The drawing under review shows one solid part. Ordinate dimensions are in mm from its lowest x, y, z. Give positions to 0.01 mm unless a question says otherwise; leave off trailing zeros. Write each loop counter-clockwise with the first axis right and the second up, starting at its lowest first coordinate (ties: lowest second). Pieces come first, ordered by that corner, then holes. Notation, with made-up numbers: (25.5, 64.5) -> (30.5, 64.5) arc R18 ccw to (30.5, 87.5) -> close; hole circle Ø5 at (28, 54.25). An arc over 180 degrees is marked (long way). Use CSV: the item, a comma, the result in double quotes.
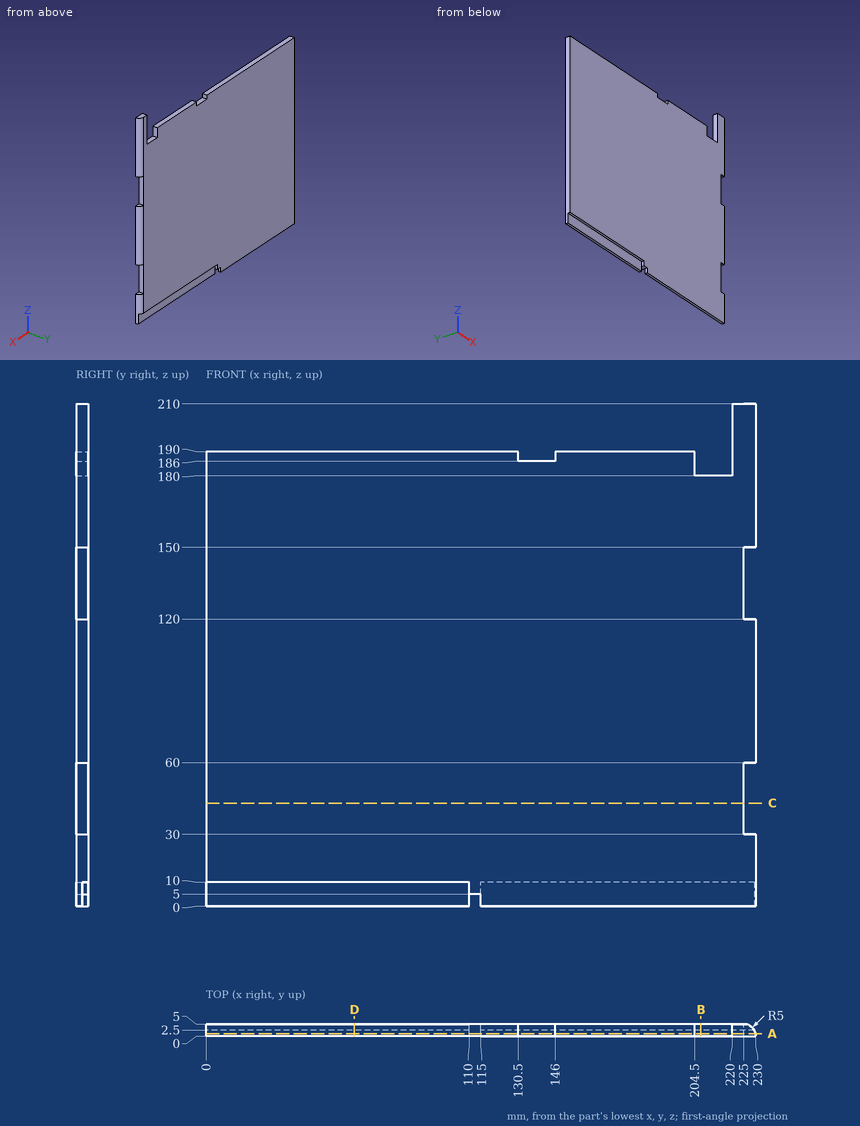
(1) Take a section at B-B (x = 207). Write out the cut boundary in (y, z), then the cut area to 3 significant figures.
Established:
outline,"(0, 0) -> (2.5, 0) -> (2.5, 10) -> (5, 10) -> (5, 180) -> (0, 180) -> close"
area,"875 mm2"
(2) Clearance check with flat-ended pins moving along their axes: pin 1 (8 mm diameter, centred on x = 132.5, z = 166, fed in from -Y); pin 2 (1 mm diameter, centred on x = 123.5, y = 1, fed in from +Z); pin 3 (2 mm diameter, centred on y = 1.5, z = 188.5, fed in from +X) (3 decimals); pin 4 (3 mm diameter, centred on x = 51.5, y = 0.5, fed in from -Z). State where each tip first meets the part, or that it passes through.
Established:
pin 1,"stops at y = 0"
pin 2,"stops at z = 190"
pin 3,"stops at x = 229.975"
pin 4,"stops at z = 10"
(3) Take a section at D-D (x = 62). Write out the cut boundary in (y, z), then the cut area to 3 significant figures.
Established:
outline,"(0, 10) -> (2.5, 10) -> (2.5, 0) -> (5, 0) -> (5, 190) -> (0, 190) -> close"
area,"925 mm2"
(4) Take a section at A-A (y = 0.95). Write out the cut boundary in (x, z), then the cut area to 3 significant figures.
Established:
outline,"(0, 10) -> (110, 10) -> (110, 5) -> (115, 5) -> (115, 0) -> (229.91, 0) -> (229.91, 30) -> (225, 30) -> (225, 60) -> (229.91, 60) -> (229.91, 120) -> (225, 120) -> (225, 150) -> (229.91, 150) -> (229.91, 210) -> (220, 210) -> (220, 180) -> (204.5, 180) -> (204.5, 190) -> (146, 190) -> (146, 186) -> (130.5, 186) -> (130.5, 190) -> (0, 190) -> close"
area,"42,200 mm2"
(5) Take a section at C-C (z = 43). Write out the cut boundary in (x, y), then the cut area to 4 significant figures.
Established:
outline,"(0, 0) -> (225, 0) -> (225, 5) -> (0, 5) -> close"
area,"1,125 mm2"
(6) For line 1 along X through (y, z) = (1.45, 189) (3 decimals); line 2 along X through (y, z) = (4.3, 120.5); line 3 along X through (y, z) = (0.25, 68.5), list the stretches that pass through material, from the lowest coordinate up. Write a range as [from, to].
Established:
line 1,"x = [0, 130.5], [146, 204.5], [220, 229.785]"
line 2,"x = [0, 225]"
line 3,"x = [0, 229.99]"
